Input: part model. Units: mm. Frame: model coordinates. Coordinates: 2 decimals unless noted, no trailing zeros. Write each loop counter-clockwise with the first axis right and the second up, starting at its lowest first coordinate (ties: lowest second). Pieces come first, ordered by that corner, then holes. Notation, with made-up numbers: (15, 18.5) - (43, 18.5) arc R28 ccw to (43, 48.5) - close; hole circle Ø2 at (11, 39). An arc over 180 degrees is marked (long way). Use CSV: the item, a comma, the result in double quotes.
```python
from build123d import *

# Parameters (mm, degrees)
SKETCH2_W           = 5
SKETCH2_H           = 82.6
SKETCH2_W_2         = 82.6
SKETCH2_H_2         = 5
BOSS_EXTRUDE1_DEPTH = 2.25
SKETCH5_R           = 1.5
CUT_EXTRUDE3_DEPTH  = 10
SKETCH6_W           = 24.487512306
SKETCH6_H           = 29.223395674
SKETCH6_H_2         = 15.523504638
SKETCH6_W_2         = 26.803129216
CUT_EXTRUDE4_DEPTH  = 10
CUT_EXTRUDE5_DEPTH  = 0.5


with BuildPart() as part:
    # Sketch2 → Boss-Extrude1 (new body)
    with BuildSketch(Plane(origin=(0, 0, 0), x_dir=(1, 0, 0), z_dir=(0, 1, 0))):
        with Locations((-43.8, 0)):
            Rectangle(SKETCH2_W, SKETCH2_H)
        Rectangle(SKETCH2_W_2, SKETCH2_H)
        with Locations((0, -43.8)):
            Rectangle(SKETCH2_W_2, SKETCH2_H_2)
        with Locations((43.8, 0)):
            Rectangle(SKETCH2_W, SKETCH2_H)
        with Locations((0, 43.8)):
            Rectangle(SKETCH2_W_2, SKETCH2_H_2)
    extrude(amount=BOSS_EXTRUDE1_DEPTH)

    # Sketch5 → Cut-Extrude3 (cut)
    with BuildSketch(Plane(origin=(0, 2.25, 0), x_dir=(1, 0, 0), z_dir=(0, 1, 0))):
        with Locations((-27.7, 35.8)):
            Circle(SKETCH5_R)
        with Locations((30.3, 35.8)):
            Circle(SKETCH5_R)
        with Locations((30.3, -13.2)):
            Circle(SKETCH5_R)
        with Locations((-27.7, -13.2)):
            Circle(SKETCH5_R)
    extrude(amount=-CUT_EXTRUDE3_DEPTH, mode=Mode.SUBTRACT)

    # Sketch6 → Cut-Extrude4 (cut)
    with BuildSketch(Plane(origin=(0, 2.25, 0), x_dir=(1, 0, 0), z_dir=(0, 1, 0))):
        with Locations((0, 22.373450156)):
            Rectangle(SKETCH6_W, SKETCH6_H)
        Rectangle(SKETCH6_W, SKETCH6_H_2)
        with Locations((25.645320761, 0)):
            Rectangle(SKETCH6_W_2, SKETCH6_H_2)
        with Locations((0, -22.373450156)):
            Rectangle(SKETCH6_W, SKETCH6_H)
        with Locations((-25.645320761, 0)):
            Rectangle(SKETCH6_W_2, SKETCH6_H_2)
    extrude(amount=-CUT_EXTRUDE4_DEPTH, mode=Mode.SUBTRACT)

    # Sketch7 → Cut-Extrude5 (cut)
    with BuildSketch(Plane(origin=(0, 2.25, 0), x_dir=(1, 0, 0), z_dir=(0, 1, 0))):
        Polygon((35.998717949, 27.449358974), (36.65, 27.449358974), (36.65, 24.111538462), (35.998717949, 24.111538462), (35.998717949, 25.495512821), (30.3, 25.495512821), (30.3, 26.065384615), (35.998717949, 26.065384615), align=None)
    extrude(amount=-CUT_EXTRUDE5_DEPTH, mode=Mode.SUBTRACT)


solid = part.part
```
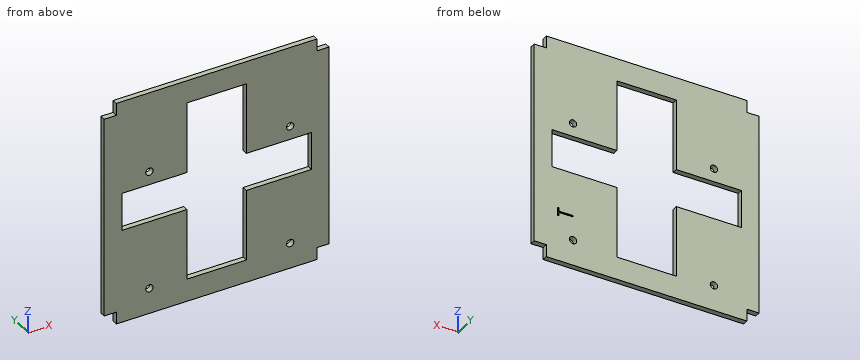
(1) Cut plane C-C on x = -27.7. Return loops of the section in (y, z).
Check values:
outline,"(0, -46.3) - (2.25, -46.3) - (2.25, -37.3) - (0, -37.3) - close; (0, -34.3) - (2.25, -34.3) - (2.25, -7.76) - (0, -7.76) - close; (0, 7.76) - (2.25, 7.76) - (2.25, 11.7) - (0, 11.7) - close; (0, 14.7) - (2.25, 14.7) - (2.25, 46.3) - (0, 46.3) - close"
(2) Cut plane D-D on z = 13.2. Return loops of the section in (x, y).
Check values:
outline,"(-46.3, 0) - (-29.2, 0) - (-29.2, 2.25) - (-46.3, 2.25) - close; (-26.2, 0) - (-12.24, 0) - (-12.24, 2.25) - (-26.2, 2.25) - close; (12.24, 0) - (28.8, 0) - (28.8, 2.25) - (12.24, 2.25) - close; (31.8, 0) - (46.3, 0) - (46.3, 2.25) - (31.8, 2.25) - close"
(3) Pin query (flat end, axial travel): pin 1 Ø2.5 at (x, z) = (30.3, 13.2) entering from -Y; pin 2 Ø0.7 at (y, z) = (1, 43) entering from +X. Return the tip coordinate at first contact, or that it passes through.
Check values:
pin 1,"through"
pin 2,"x = 41.3"
(4) Ray query, probe 1 along X at (y, z) = (1.05, 13.2); probe 2 along Z at (x, y) = (-27.7, 1.55); probe 3 along X at (y, z) = (2, -26). Return the intervals inside material, ascending. Write a range as from..to.
Check values:
probe 1,"-46.3..-29.2, -26.2..-12.24, 12.24..28.8, 31.8..46.3"
probe 2,"-46.3..-37.3, -34.3..-7.76, 7.76..11.7, 14.7..46.3"
probe 3,"-46.3..-12.24, 12.24..30.3, 36.65..46.3"
(5) Cut plane A-A on x = -4.5. Return loops of the section in (y, z).
Check values:
outline,"(0, -46.3) - (2.25, -46.3) - (2.25, -36.99) - (0, -36.99) - close; (0, 36.99) - (2.25, 36.99) - (2.25, 46.3) - (0, 46.3) - close"
(6) Cut plane B-B on z = 24. Return loops of the section in (x, y), and give its area (3 significant figures).
Check values:
outline,"(-46.3, 0) - (-12.24, 0) - (-12.24, 2.25) - (-46.3, 2.25) - close; (12.24, 0) - (46.3, 0) - (46.3, 2.25) - (12.24, 2.25) - close"
area,"153 mm^2"
